from build123d import *

# Parameters (mm, degrees)
ESBO_O2_R = 3


with BuildPart() as part:
    # Varredura1: sweep along a path in Esboço1
    with BuildLine(Plane.XY) as varredura1_path:
        Line((-22, 41.023088741), (29, 41.023088741))
        ThreePointArc((29, 41.023088741), (33.242640687, 39.265729428), (35, 35.023088741))
        Line((35, 35.023088741), (35, -82.976911259))
        ThreePointArc((35, -82.976911259), (33.242640687, -87.219551946), (29, -88.976911259))
        Line((29, -88.976911259), (-29, -88.976911259))
        ThreePointArc((-29, -88.976911259), (-33.242640687, -87.219551946), (-35, -82.976911259))
        Line((-35, -82.976911259), (-35, 35.023088741))
        ThreePointArc((-35, 35.023088741), (-33.242640687, 39.265729428), (-29, 41.023088741))
        Line((-29, 41.023088741), (-27, 41.023088741))
    # Esboço2 → Varredura1 (sweep)
    with BuildSketch(Plane(origin=(-22, 41.023088741, 0), x_dir=(0, 0, -1), z_dir=(1, 0, 0))):
        Circle(ESBO_O2_R)
    sweep(path=varredura1_path.line)


solid = part.part
The listing builds one solid part. Answer for the finished solid, in the listing's coordinates (mm). A direction names the side the tool comes from. Coordinates: 2 decimals unless noted, no trailing zeros. Write each loop counter-clockwise with the first axis right and the second up, starting at its lowest first coordinate (ties: lowest second). Pieces come first, ordered by that corner, then holes. Notation, with made-up numbers: (-9.5, -8.5) - (28.5, -8.5) arc R26 ccw to (28.5, 7.5) - close; hole circle Ø4 at (-12, 28). An arc over 180 degrees is marked (long way). Put each result on its own line as item: value.
1. The part is cut by section B-B on z = 0. Give the vertices of the cut face in (x, y), plus the area to 3 significant figures.
Answer sheet:
outline: (-38, -82.98) arc R9 ccw to (-29, -91.98) - (29, -91.98) arc R9 ccw to (38, -82.98) - (38, 35.02) arc R9 ccw to (29, 44.02) - (-22, 44.02) - (-22, 38.02) - (29, 38.02) arc R3 cw to (32, 35.02) - (32, -82.98) arc R3 cw to (29, -85.98) - (-29, -85.98) arc R3 cw to (-32, -82.98) - (-32, 35.02) arc R3 cw to (-29, 38.02) - (-27, 38.02) - (-27, 44.02) - (-29, 44.02) arc R9 ccw to (-38, 35.02) - close
area: 2,310 mm^2
2. Flat-ended cylindrical pins translate along their axes: pin 1 Ø1.8 at (y, z) = (40.5, 1) entering from +X; pin 2 Ø1 at (x, z) = (20.5, -1) entering from +Y; pin 3 Ø2 at (x, z) = (-13, -2) entering from -Y. Find the tip coordinate at first contact, or state that the pin passes through.
Answer sheet:
pin 1: stops at x = 36.62
pin 2: stops at y = 43.98
pin 3: stops at y = -91.81
3. Find the intervals of material crossed by line 1 along X through (y, z) = (-45.5, 0.5); line 2 along X through (y, z) = (18.5, 2); line 3 along Y through (x, z) = (-14, 0), in increasing order. Write a range as from..to.
Answer sheet:
line 1: x = -37.96..-32.04, 32.04..37.96
line 2: x = -37.24..-32.76, 32.76..37.24
line 3: y = -91.98..-85.98, 38.02..44.02
4. Determine the mould class of faces 3 (the face through (-22, 41, 0)), 4 (the face through (38, -25, 0)) for opening direction Y: pulls with the +Y half, pulls with the -Y half, needs draft (parallel to the pull), parting line crosses it, or undercut.
Answer sheet:
face 3: needs draft
face 4: undercut
5. A tool of negligible diameter and unlimited length cuts with its end or side. For faces 1 (the face through (-27.986, 43.553, -1.613)), 2 (the face through (-27, 41, 0)), from which of +Z, -Z, +X, -X, +Y, -Y can it reach the whole face along a straight path? Write none if from no direction.
Answer sheet:
face 1: none
face 2: +Z, -Z, +Y
6. The part is cut by section C-C on x = 23. Give the vertices of the cut face in (y, z).
Answer sheet:
outline: circle Ø6 at (-88.98, 0); circle Ø6 at (41.02, 0)
7. The part is cut by section A-A on y = -14.5. Give the vertices of the cut face in (x, z), plus the area to 3 significant figures.
Answer sheet:
outline: circle Ø6 at (-35, 0); circle Ø6 at (35, 0)
area: 56.5 mm^2
